Input: part model. Units: mm. Frame: model coordinates. Coordinates: 2 decimals unless noted, no trailing zeros. Write each loop counter-clockwise with the first axis right and the second up, starting at its lowest first coordinate (ties: lowest second). Pieces come first, ordered by that corner, then holes. Notation, with made-up numbers: M 85,79.5 L 138,79.5 A14 cw 138,92.5 Z; hole C -7,81 d4. An arc over 180 degrees is marked long. Use CSV: the item, a comma, the result in double quotes.
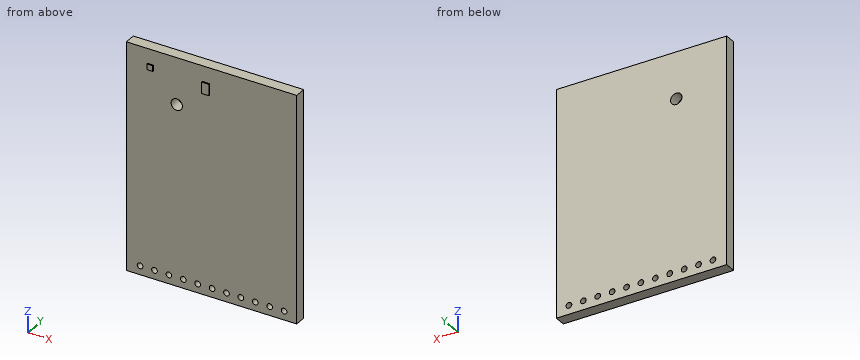
```python
from build123d import *

# Parameters (mm, degrees)
SKETCH1_W           = 30.06
SKETCH1_H           = 2
BOSS_EXTRUDE1_DEPTH = 39.95
SKETCH2_R           = 1
CUT_EXTRUDE1_DEPTH  = 39.95
SKETCH3_R           = 0.5
CUT_EXTRUDE2_DEPTH  = 4.5
LPATTERN1_COUNT     = 11
LPATTERN1_PITCH     = 2.54
SKETCH4_W           = 1.3
SKETCH4_H           = 2
BOSS_EXTRUDE2_DEPTH = 0.2
SKETCH5_W           = 1
SKETCH5_H           = 1
BOSS_EXTRUDE3_DEPTH = 0.2


with BuildPart() as part:
    # Sketch1 → Boss-Extrude1 (new body)
    with BuildSketch(Plane.XY):
        with Locations((15.03, 1)):
            Rectangle(SKETCH1_W, SKETCH1_H)
    extrude(amount=BOSS_EXTRUDE1_DEPTH)

    # Sketch2 → Cut-Extrude1 (cut)
    with BuildSketch(Plane(origin=(0, 2, 0), x_dir=(1, 0, 0), z_dir=(0, 1, 0))):
        with Locations(Location((8.9, -31.75, 0), (0, 0, 270))):
            Circle(SKETCH2_R)
    extrude(amount=-CUT_EXTRUDE1_DEPTH, mode=Mode.SUBTRACT)

    # Sketch3 → Cut-Extrude2 (cut)
    with BuildSketch(Plane(origin=(0, 2, 0), x_dir=(1, 0, 0), z_dir=(0, 1, 0))):
        with Locations(Location((27.83, -1.56, 0), (0, 0, 270))):
            Circle(SKETCH3_R)
    cut_extrude2 = extrude(amount=-CUT_EXTRUDE2_DEPTH, mode=Mode.SUBTRACT)

    # LPattern1: Cut-Extrude2 ×11
    with Locations(*[(-i * LPATTERN1_PITCH, 0, 0) for i in range(1, LPATTERN1_COUNT)]):
        add(cut_extrude2, mode=Mode.SUBTRACT)

    # Sketch4 → Boss-Extrude2 (add)
    with BuildSketch(Plane.XZ):
        with Locations((14.06, 36.2)):
            Rectangle(SKETCH4_W, SKETCH4_H)
    extrude(amount=BOSS_EXTRUDE2_DEPTH)

    # Sketch5 → Boss-Extrude3 (add)
    with BuildSketch(Plane.XZ):
        with Locations((4.26, 36.86)):
            Rectangle(SKETCH5_W, SKETCH5_H)
    extrude(amount=BOSS_EXTRUDE3_DEPTH)


solid = part.part
```
1. Section B-B (z = 27). Return loops of the section in (x, y).
Resolved:
outline,"M 0,0 L 30.06,0 L 30.06,2 L 0,2 Z"
2. Material intervals for line 1 (Z direction, x = 12.59, y = 0.65); line 2 (Y direction, x = 19, z = 30); line 3 (Z direction, x = 23, y = 0.4), sorted ascending. Write a range as [from, to].
Resolved:
line 1,"z = [0, 1.06], [2.06, 39.95]"
line 2,"y = [0, 2]"
line 3,"z = [0, 1.13], [1.99, 39.95]"
3. Contact query for flat-ended pins moving along their axis: pin 1 Ø6 at (x, z) = (16, 17) entering from -Y; pin 2 Ø1.8 at (x, z) = (8.9, 31.75) entering from +Y. Output: stop coordinate, or through.
Resolved:
pin 1,"stops at y = 0"
pin 2,"passes through"
4. Section A-A (x = 17.67). Return loops of the section in (y, z), then the cut area to 3 significant figures.
Resolved:
outline,"M 0,0 L 2,0 L 2,1.06 L 0,1.06 Z; M 0,2.06 L 2,2.06 L 2,39.95 L 0,39.95 Z"
area,"77.9 mm^2"
